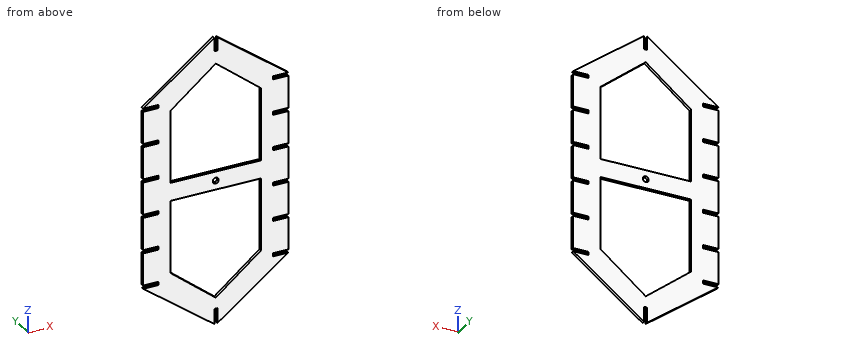
from build123d import *

# Parameters (mm, degrees)
BOSS_EXTRUDE1_DEPTH = 3.175
SKETCH3_R           = 3.25
SKETCH3_W           = 17
SKETCH3_H           = 3.5
CUT_EXTRUDE1_DEPTH  = 4.175
SKETCH4_W           = 3.5
SKETCH4_H           = 18
SKETCH4_H_2         = 16
CUT_EXTRUDE2_DEPTH  = 4.175


with BuildPart() as part:
    # Sketch2 → Boss-Extrude1 (new body)
    with BuildSketch(Plane(origin=(0, 0, 0), x_dir=(1, 0, 0), z_dir=(0, 1, 0))):
        Polygon((0, 200), (80, 260), (160, 200), (160, 0), (80, -60), (0, 0), align=None)
    extrude(amount=BOSS_EXTRUDE1_DEPTH)

    # Sketch3 → Cut-Extrude1 (cut, through all)
    with BuildSketch(Plane(origin=(0, 3.175, 0), x_dir=(1, 0, 0), z_dir=(0, 1, 0))):
        with Locations((80, 100)):
            Circle(SKETCH3_R)
        Polygon((30, 190), (80, 230), (130, 190), (130, 110), (30, 110), align=None)
        with Locations((8.5, 158.95)):
            Rectangle(SKETCH3_W, SKETCH3_H)
        Polygon((30, 90), (30, 10), (80, -30), (130, 10), (130, 90), align=None)
        with Locations((8.5, 198.25)):
            Rectangle(SKETCH3_W, SKETCH3_H)
        with Locations((8.5, 119.65)):
            Rectangle(SKETCH3_W, SKETCH3_H)
        with Locations((8.5, 80.35)):
            Rectangle(SKETCH3_W, SKETCH3_H)
        with Locations((8.5, 41.05)):
            Rectangle(SKETCH3_W, SKETCH3_H)
        with Locations((8.5, 1.75)):
            Rectangle(SKETCH3_W, SKETCH3_H)
        with Locations((151.5, 1.75)):
            Rectangle(SKETCH3_W, SKETCH3_H)
        with Locations((151.5, 41.05)):
            Rectangle(SKETCH3_W, SKETCH3_H)
        with Locations((151.5, 80.35)):
            Rectangle(SKETCH3_W, SKETCH3_H)
        with Locations((151.5, 119.65)):
            Rectangle(SKETCH3_W, SKETCH3_H)
        with Locations((151.5, 158.95)):
            Rectangle(SKETCH3_W, SKETCH3_H)
        with Locations((151.5, 198.25)):
            Rectangle(SKETCH3_W, SKETCH3_H)
    extrude(amount=-CUT_EXTRUDE1_DEPTH, mode=Mode.SUBTRACT)

    # Sketch4 → Cut-Extrude2 (cut, through all)
    with BuildSketch(Plane(origin=(0, 3.175, 0), x_dir=(1, 0, 0), z_dir=(0, 1, 0))):
        with Locations((80.16, 251)):
            Rectangle(SKETCH4_W, SKETCH4_H)
        with Locations((80.16, -52)):
            Rectangle(SKETCH4_W, SKETCH4_H_2)
    extrude(amount=-CUT_EXTRUDE2_DEPTH, mode=Mode.SUBTRACT)


solid = part.part
Read the model definition and answer for the solid it produces. Units are mm, in the model's axes. Give positions to 0.01 mm unless a question says otherwise; leave off trailing zeros. Loops run counter-clockwise (first coordinate to the right, second up) from the corner with the lowest first, then second, coordinate; pieces in that order, holes last. Notation, with made-up numbers: (21.25, 75) -> (42.25, 75) arc R18 cw to (42.25, 92) -> close; hole circle Ø6 at (-4, 54.25). An arc over 180 degrees is marked (long way). Use a Markdown table: item, result.
Q1. Section C-C, the plane x = 115 is taken. Determine the outline of the cut face in (y, z) (3 decimals), then the cut area to 3 significant figures.
Solved:
| item | result |
|---|---|
| outline | (0, -233.75) -> (3.175, -233.75) -> (3.175, -202) -> (0, -202) -> close; (0, -110) -> (3.175, -110) -> (3.175, -90) -> (0, -90) -> close; (0, 2) -> (3.175, 2) -> (3.175, 33.75) -> (0, 33.75) -> close |
| area | 265 mm^2 |
Q2. Section A-A, the plane x = 59 is taken. Determine the outline of the cut face in (y, z) (3 decimals).
Solved:
| item | result |
|---|---|
| outline | (0, -244.25) -> (3.175, -244.25) -> (3.175, -213.2) -> (0, -213.2) -> close; (0, -110) -> (3.175, -110) -> (3.175, -90) -> (0, -90) -> close; (0, 13.2) -> (3.175, 13.2) -> (3.175, 44.25) -> (0, 44.25) -> close |
Q3. Section B-B, the plane z = -144 is taken. Determine the outline of the cut face in (x, y) (3 decimals), then the cut area to 4 significant figures.
Solved:
| item | result |
|---|---|
| outline | (0, 0) -> (30, 0) -> (30, 3.175) -> (0, 3.175) -> close; (130, 0) -> (160, 0) -> (160, 3.175) -> (130, 3.175) -> close |
| area | 190.5 mm^2 |
Q4. Each of these flat-tipped pins is pushed along its axis until it touches: pin 1 (1 mm diameter, centred on x = 94.5, y = 1, fed in from +Z); pin 2 (1.6 mm diameter, centred on x = 7.5, y = 1.5, fed in from +Z) (3 decimals); pin 3 (1.6 mm diameter, centred on x = 10.5, y = 1, fed in from +Z) (3 decimals); pin 4 (1.5 mm diameter, centred on y = 1.5, z = -189.5, fed in from -X). Where does it stop, or does it pass through?
Solved:
| item | result |
|---|---|
| pin 1 | stops at z = 49.5 |
| pin 2 | stops at z = 6.225 |
| pin 3 | stops at z = 8.475 |
| pin 4 | stops at x = 0 |
Q5. Find the intervals of material crossed by line 1 along Z through (x, y) = (80, 2.4); line 2 along X through (y, z) = (1.05, -100); line 3 along X through (y, z) = (2.45, -122), in increasing order.
Solved:
| item | result |
|---|---|
| line 1 | z = -242 to -230, -110 to -103.25, -96.75 to -90, 30 to 44 |
| line 2 | x = 0 to 76.75, 83.25 to 160 |
| line 3 | x = 0 to 30, 130 to 160 |
Q6. Section D-D, the plane y = 1.2 is taken. Count the separate pieces of the cut face and the enclosed holes in it, then the cut area to 3 significant figures.
Solved:
| item | result |
|---|---|
| separate pieces | 1 |
| enclosed holes | 3 |
| area | 20,700 mm^2 |
